Input: part model. Units: mm. Frame: model coordinates. A direction names the side the tool comes from. Coordinates: 2 decimals unless noted, no trailing zeros. Order: outer loops, then holes, each group sorted by start corner. A loop starts at its lowest first (then second) coordinate and runs counter-clockwise, first axis right, second up.
Autodesk Inventor part; units mm, degrees
ref_plane "YZ Plane" through (0, 0, 0) normal (1, 0, 0) x (0, 1, 0)
ref_plane "XZ Plane" through (0, 0, 0) normal (0, 1, 0) x (-1, 0, 0)
ref_plane "XY Plane" through (0, 0, 0) normal (0, 0, 1) x (1, 0, 0)
sketch "Sketch1" plane through (0, 0, 0) normal (0, 0, 1) x (1, 0, 0)
  line L0 (0, -28.7085) -> (0, 28.7085)
  line L1 (0, 28.7085) -> (0, -28.7085)
  line L2 (-38.5085, 0) -> (38.5085, 0)
  line L3 (0, -16.2635) -> (16.2635, 0)
  line L4 (16.2635, 0) -> (0, 16.2635)
  line L5 (0, 16.2635) -> (-16.2635, 0)
  line L6 (-16.2635, 0) -> (0, -16.2635)
  line L7 (0, -16.2635) -> (0, 16.2635) construction
  line L8 (16.2635, 0) -> (-16.2635, 0) construction
  line L9 (0, -16.2635) -> (23, -16.2635) construction
  line L10 (0, -20.5061) -> (-17.5061, -3)
  line L11 (-17.5061, -3) -> (-27.5061, -3)
  line L12 (-27.5061, -3) -> (-27.5061, 3)
  line L13 (-27.5061, 3) -> (-17.5061, 3)
  line L14 (-17.5061, 3) -> (0, 20.5061)
  line L15 (0, 20.5061) -> (17.5061, 3)
  line L16 (17.5061, -3) -> (0, -20.5061)
  line L17 (-38.5085, 0) -> (38.5085, 0)
  line L18 (-27.5061, 0) -> (-16.2635, 0)
  line L19 (16.2635, 0) -> (23.5061, 0)
  line L20 (17.5061, -3) -> (27.5061, -3)
  line L21 (27.5061, -3) -> (27.5061, 3)
  line L22 (27.5061, 3) -> (17.5061, 3)
  line L23 (16.2635, 0) -> (27.5061, 0)
  point P0 (0, 0)
  point P1 (-16.2635, 0)
  point P2 (16.2635, 0)
  point P3 (27.5061, 0)
  dimension "d34" = 23
  dimension "d35" = 45
  dimension "d36" = 23
  dimension "d37" = 3
  dimension "d38" = 3
  dimension "d39" = 45
  dimension "d41" = 6
  dimension "d49" = 10
  dimension "d50" = 6
  dimension "d51" = 3
  dimension "d52" = 10
extrude "Extrusion2" add sketch "Sketch1" along normal blind 24 contours L4 L0 L15 L22 L21 L2 | L2 L12 L13 L14 L0 L5
sketch "Sketch3" plane through (-27.5061, 3, 0) normal (0, 1, 0) x (1, 0, 0)
  line L0 (66.0146, 0) -> (-11.0024, 0)
  line L1 (0, 0) -> (0, -24)
  line L2 (55.0122, 0) -> (55.0122, -24)
  point P0 (27.5061, 0)
  point P1 (5, -12)
  point P2 (50.0122, -12)
  dimension "d55" = 12
  dimension "d56" = 12
  dimension "d57" = 5
  dimension "d58" = 5
hole "Hole1" at (-22.5061, 3, 12) at (22.5061, 3, 12) direction (0, -1, 0) diameter 4 end through all
chamfer "Chamfer1" distance 2 angle 45 2 edges at (0, 20.5061, 12) (0, 16.2635, 12)
properties part number "Fan_top_3DPrint"
Item 1: Draft query along Z for faces 4 (the face through (-6.2, 10.3, 0)), 5 (the face through (23.72, 1.48, 10.41)), 6 (the face through (-25, 3, 12)). Return one class per face: pulls with the +Z half, pulls with the -Z half, needs draft (parallel to the pull), parting line crosses it, or undercut.
Response values:
face 4: pulls with the -Z half
face 5: undercut
face 6: needs draft
Item 2: Cut plane A-A on z = 12. Return loops of the section in (x, y).
Response values:
outline: (-27.51, 0) - (-24.51, 0) - (-24.51, 3) - (-27.51, 3) - close; (-20.51, 0) - (-16.26, 0) - (-1.41, 14.85) - (1.41, 14.85) - (16.26, 0) - (20.51, 0) - (20.51, 3) - (17.51, 3) - (1.41, 19.09) - (-1.41, 19.09) - (-17.51, 3) - (-20.51, 3) - close; (24.51, 0) - (27.51, 0) - (27.51, 3) - (24.51, 3) - close
Item 3: Cut plane D-D on x = 14. Return loops of the section in (y, z).
Response values:
outline: (2.26, 0) - (6.51, 0) - (6.51, 24) - (2.26, 24) - close
Item 4: Cut plane B-B on z = 14.75. Return loops of the section in (x, y).
Response values:
outline: (-27.51, 0) - (-16.26, 0) - (-1.41, 14.85) - (1.41, 14.85) - (16.26, 0) - (27.51, 0) - (27.51, 3) - (17.51, 3) - (1.41, 19.09) - (-1.41, 19.09) - (-17.51, 3) - (-27.51, 3) - close
Item 5: Access query for faces 1 (the face through (25, 3, 12)), 2 (the face through (19, 0, 12)), 3 (the face through (0, 14.849, 12)). Directions: +Z, -Z, +X, -X, +Y, -Y. A direction counts if a zero-diameter tool reaches every point of the face in a straight line with its end or side. Return the directions, or none.
Response values:
face 1: +Z, -Z, +X, +Y
face 2: +Z, -Z, +X, -X, -Y
face 3: +Z, -Z, -Y
Item 6: Pin query (flat end, axial travel): pin 1 Ø11 at (x, z) = (21, 16) entering from +Y; pin 2 Ø3 at (x, z) = (-20.5, 11.5) entering from +Y; pin 3 Ø4 at (x, z) = (-9.5, 7.5) entering from -Y; pin 4 Ø3.5 at (x, z) = (-22.51, 12) entering from +Y. Return the tip coordinate at first contact, or that it passes through.
Response values:
pin 1: stops at y = 5.01
pin 2: stops at y = 3
pin 3: stops at y = 4.76
pin 4: passes through
Item 7: Cut plane C-C on y = 16. Return loops of the section in (x, z).
Response values:
outline: (-4.51, 0) - (4.51, 0) - (4.51, 24) - (-4.51, 24) - close
Item 8: Ray query, probe 1 along X at (y, z) = (1.3, 12); probe 2 along X at (y, z) = (1.2, 12); probe 3 along X at (y, z) = (1.5, 8.5). Return the intervals inside material, ascending.
Response values:
probe 1: x = -27.51 to -24.51, -20.51 to -14.96, 14.96 to 20.51, 24.51 to 27.51
probe 2: x = -27.51 to -24.51, -20.51 to -15.06, 15.06 to 20.51, 24.51 to 27.51
probe 3: x = -27.51 to -14.76, 14.76 to 27.51
